Model file for the job. Use its own axes, mm. Face numbers are marked on the shaded views. A direction names the side the tool comes from. Coordinates: 2 decimals unless noted, no trailing zeros. Order: outer loops, then holes, each group sorted by start corner. A loop starts at its lowest first (then second) coordinate and runs counter-clockwise, first axis right, second up.
from build123d import *

# Parameters (mm, degrees)
F0_W      = 1550.9875
F0_H      = 25.4
F1_DEPTH  = 174.625
F3_W      = 1419.225
F3_H      = 25.4
F4_DEPTH  = 130.175
F5_W      = 1292.225
F5_H      = 25.4
F6_DEPTH  = 73.025
F2_W      = 1363.6625
F2_H      = 250.825
F7_DEPTH  = 25.4
F9_DEPTH  = 12.7
F10_W     = 936.912687
F10_H     = 531.850287
F11_DEPTH = 174.626
F13_DEPTH = 174.626


with BuildPart() as f1:
    # F0 (on Front) → F1 (new body)
    with BuildSketch(Plane.XZ):
        with Locations((0, -12.7)):
            Rectangle(F0_W, F0_H)
    extrude(amount=F1_DEPTH)

    # F3 (on Front) → F4 (join)
    with BuildSketch(Plane.XZ):
        with Locations((0, -38.1)):
            Rectangle(F3_W, F3_H)
    extrude(amount=F4_DEPTH)

    # F5 (on Front) → F6 (join)
    with BuildSketch(Plane.XZ):
        with Locations((0, -63.5)):
            Rectangle(F5_W, F5_H)
    extrude(amount=F6_DEPTH)

    # F2 (on Front) → F7 (join)
    with BuildSketch(Plane.XZ):
        with Locations((7.9375, -150.8125)):
            Rectangle(F2_W, F2_H)
    extrude(amount=F7_DEPTH)

    # F8 (on face) → F9 (cut)
    with BuildSketch(Plane.XZ.offset(25.4)):
        Polygon((-673.89375, -50.8), (-673.89375, -276.225), (-620.7125, -276.225), (-620.7125, -76.2), (-646.1125, -76.2), (-646.1125, -50.8), align=None)
        Polygon((620.7125, -76.2), (620.7125, -276.225), (689.76875, -276.225), (689.76875, -50.8), (646.1125, -50.8), (646.1125, -76.2), align=None)
    extrude(amount=-F9_DEPTH, mode=Mode.SUBTRACT)

    # F10 (on Front) → F11 (cut, through all)
    with BuildSketch(Plane.XZ):
        with Locations((-380.350093, -119.809725)):
            Rectangle(F10_W, F10_H)
    extrude(amount=F11_DEPTH, mode=Mode.SUBTRACT)

    # F12 (on Front) → F13 (cut, through all)
    with BuildSketch(Plane.XZ):
        Polygon((237.33125, -25.4), (237.33125, 0), (148.372248, 68.829454), (-112.537719, 31.016426), (38.714431, -95.657267), (88.10625, -76.2), (135.73125, -76.2), (135.73125, -50.8), (192.88125, -50.8), (192.88125, -25.4), align=None)
    extrude(amount=F13_DEPTH, mode=Mode.SUBTRACT)


solid = f1.part
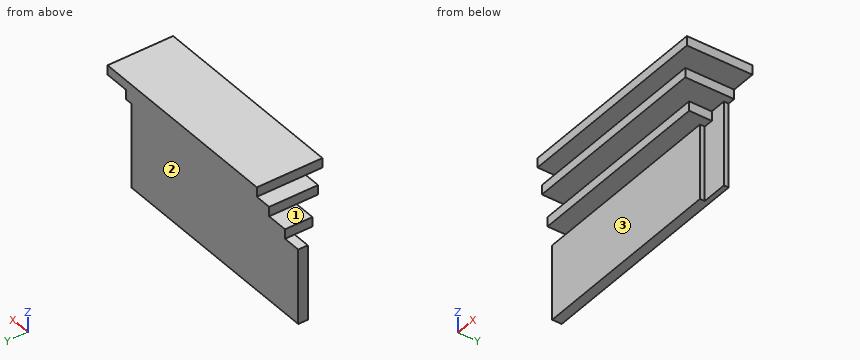
Q1. Drop flat-ended pins along their axis: P1, Ø12.5, axis at y = -88, z = -40, coming from the +X side; P2, Ø2, axis at x = 200.5, z = -247.5, coming from the -Y side; P3, Ø20.5, axis at y = -47.5, z = -63.5, coming from the +X side. Give the stop position or say it passes through.
Established:
P1: stops at x = 709.61
P2: stops at y = -25.4
P3: stops at x = 646.11
Q2. Which spindle directions (+Z, -Z, +X, -X, +Y, -Y) get a long thin tool onto all of the face, cutting with end or side? Do the marked faces 1, 2 and 3. Say none if no direction does.
Established:
face 1: +Z, -X, +Y, -Y
face 2: +Z, -Z, +X, -X, +Y
face 3: -Z, +X, -X, -Y
Q3. Cut at B-B, the plane y = -52. List the corners of the cut face in (x, z).
Established:
outline: (135.73, -76.2) - (646.11, -76.2) - (646.11, -50.8) - (709.61, -50.8) - (709.61, -25.4) - (775.49, -25.4) - (775.49, 0) - (237.33, 0) - (237.33, -25.4) - (192.88, -25.4) - (192.88, -50.8) - (135.73, -50.8) - close
Q4. Cut at A-A, the plane x = 201. List the corners of the cut face in (y, z) (3 decimals), plus the area to 3 significant figures.
Established:
outline: (-130.175, -50.8) - (-73.025, -50.8) - (-73.025, -76.2) - (-25.4, -76.2) - (-25.4, -276.225) - (0, -276.225) - (0, -25.4) - (-130.175, -25.4) - close
area: 10,200 mm2
Q5. Cut at D-D, the plane y = -82.5. List the corners of the cut face in (x, z), plus the area to 3 significant figures.
Established:
outline: (192.88, -50.8) - (709.61, -50.8) - (709.61, -25.4) - (775.49, -25.4) - (775.49, 0) - (237.33, 0) - (237.33, -25.4) - (192.88, -25.4) - close
area: 26,800 mm2
Q6. Probe line 1 (Z direction, x = 327.5, y = -70); line 2 (X direction, y = -14.5, z = -182); line 3 (Y direction, x = 313, z = -54) (3 decimals). List the from-to ranges inside material, lowest first.
Established:
line 1: z = -76.2 to 0
line 2: x = 88.11 to 620.71
line 3: y = -73.025 to 0
Q7. Cut at C-C, the plane z = -190. List the corners of the cut face in (x, y), plus the area to 3 significant figures.
Established:
outline: (88.11, -25.4) - (620.71, -25.4) - (620.71, -12.7) - (689.77, -12.7) - (689.77, 0) - (88.11, 0) - close
area: 14,400 mm2
